Geometry check sheet. Reference: the model listing, model coordinates, mm. Face numbers are marked on the shaded views. Round coordinates to 2 decimals unless told otherwise and drop trailing zeros. Loops run counter-clockwise (first coordinate to the right, second up) from the corner with the lowest first, then second, coordinate; pieces in that order, holes last. Notation, with made-up numbers: (86, 36) - (139, 36) arc R12 cw to (139, 50) - close; hole circle Ø3 at (-28, 7). An arc over 180 degrees is marked (long way). Answer as CSV lines item,"result". Start each with the question number.
1) Cross-section at B-B on z = 2.1. Record the boundary of the cut face in (x, y), and give its area (3 significant figures).
2) Thickness scan on line 1 along Y through (x, z) = (-0.5, 1.65); line 2 along Z through (x, y) = (1, -3.5); line 3 along X through (y, z) = (-2.5, 1.75). Record the ranges inside material, lowest first.
3) Depth check by flat-ended pin: P1, Ø1.3, axis at y = 7.5, z = 2, coming from the +X side; P2, Ø0.7, axis at x = 2.5, y = 6, coming from the +Z side; P3, Ø0.5, axis at y = 10.5, z = 2, coming from the +X side. Enter the tip coordinate at first touch or a pass-through.
4) Draft check along Y on the marked faces 1, 2, 3 and 4. Enter one of: released by +Y, released by -Y, zero draft, split by the parting line, or undercut.
5) Cross-section at A-A on x = 0.5. Record the boundary of the cut face in (y, z).
6) Cross-section at D-D on y = -8.5. Record the boundary of the cut face in (x, z), and give its area (3 significant figures).
7) Cross-section at C-C on x = 2. Record the boundary of the cut face in (y, z), and give its area (3 significant figures).
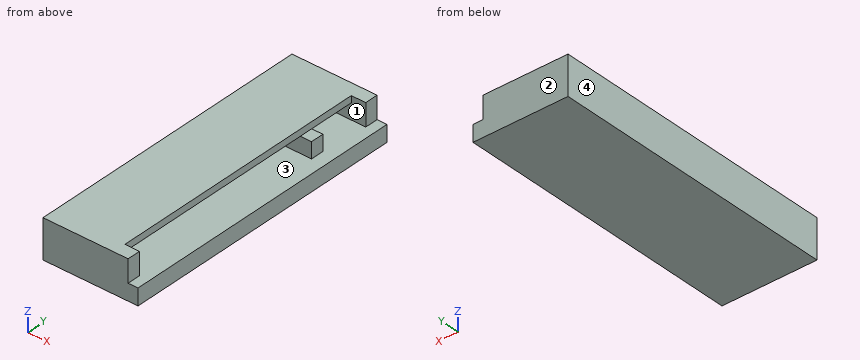
from build123d import *

# Parameters (mm, degrees)
SKETCH009_W   = 7.2
SKETCH009_H   = 22
PAD006_DEPTH  = 1.25
SKETCH010_W   = 1
SKETCH010_H   = 22
SKETCH010_W_2 = 5.45
SKETCH010_H_2 = 1
SKETCH010_W_3 = 5.2
PAD007_DEPTH  = 1.2
SKETCH011_W   = 5.35
SKETCH011_H   = 22
SKETCH011_W_2 = 1.1
SKETCH011_H_2 = 1
PAD008_DEPTH  = 0.5


with BuildPart() as part:
    # Sketch009 → Pad006 (new body)
    with BuildSketch(Plane.XY):
        Rectangle(SKETCH009_W, SKETCH009_H)
    extrude(amount=PAD006_DEPTH)

    # Sketch010 (on Face6 of Pad006) → Pad007 (join)
    with BuildSketch(Plane.XY.offset(1.25)):
        with Locations((-3.1, 0)):
            Rectangle(SKETCH010_W, SKETCH010_H)
        with Locations((0.125, 10.5)):
            Rectangle(SKETCH010_W_2, SKETCH010_H_2)
        with Locations((0, 6)):
            Rectangle(SKETCH010_W_3, SKETCH010_H_2)
        with Locations((0.125, -10.5)):
            Rectangle(SKETCH010_W_2, SKETCH010_H_2)
    extrude(amount=PAD007_DEPTH)

    # Sketch011 (on Face16 of Pad007) → Pad008 (join)
    with BuildSketch(Plane.XY.offset(2.45)):
        with Locations((-0.925, 0)):
            Rectangle(SKETCH011_W, SKETCH011_H)
        with Locations((2.3, -10.5)):
            Rectangle(SKETCH011_W_2, SKETCH011_H_2)
        with Locations((2.3, 10.5)):
            Rectangle(SKETCH011_W_2, SKETCH011_H_2)
    extrude(amount=PAD008_DEPTH)


solid = part.part
Answer block:
1,outline,"(-3.6, -11) - (2.85, -11) - (2.85, -10) - (-2.6, -10) - (-2.6, 5.5) - (2.6, 5.5) - (2.6, 6.5) - (-2.6, 6.5) - (-2.6, 10) - (2.85, 10) - (2.85, 11) - (-3.6, 11) - close"
1,area,"38.1 mm^2"
2,line 1,"y = -11 to -10, 5.5 to 6.5, 10 to 11"
2,line 2,"z = 0 to 1.25, 2.45 to 2.95"
2,line 3,"x = -3.6 to -2.6"
3,P1,"stops at x = 1.75"
3,P2,"stops at z = 2.45"
3,P3,"stops at x = 2.85"
4,face 1,"undercut"
4,face 2,"released by +Y"
4,face 3,"undercut"
4,face 4,"zero draft"
5,outline,"(-11, 0) - (11, 0) - (11, 2.95) - (-11, 2.95) - close; hole (-10, 1.25) - (5.5, 1.25) - (5.5, 2.45) - (-10, 2.45) - close; hole (6.5, 1.25) - (10, 1.25) - (10, 2.45) - (6.5, 2.45) - close"
6,outline,"(-3.6, 0) - (3.6, 0) - (3.6, 1.25) - (-2.6, 1.25) - (-2.6, 2.45) - (1.75, 2.45) - (1.75, 2.95) - (-3.6, 2.95) - close"
6,area,"12.9 mm^2"
7,outline,"(-11, 0) - (11, 0) - (11, 2.95) - (10, 2.95) - (10, 1.25) - (6.5, 1.25) - (6.5, 2.45) - (5.5, 2.45) - (5.5, 1.25) - (-10, 1.25) - (-10, 2.95) - (-11, 2.95) - close"
7,area,"32.1 mm^2"
